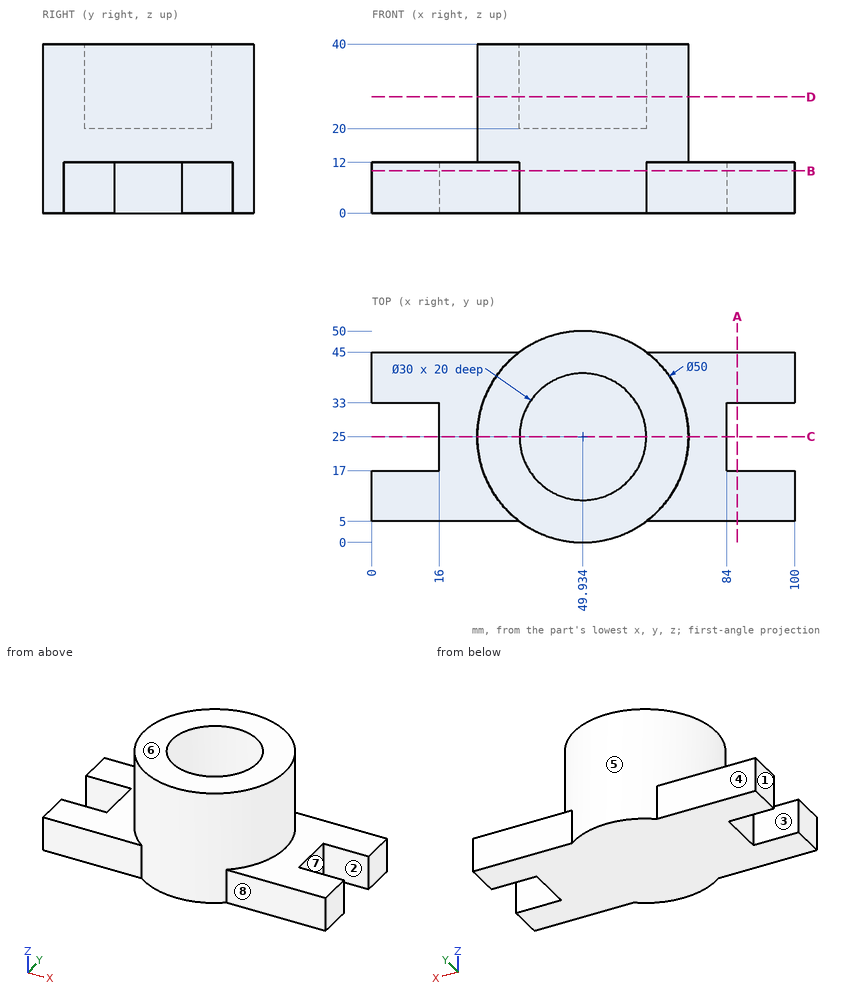
Check sheet for the drawn part. Datum: minimum x, y, z corner. Units: mm. A direction names the side the tool comes from. Coordinates: 2 decimals unless noted, no trailing zeros. Loops run counter-clockwise (first coordinate to the right, second up) from the corner with the lowest first, then second, coordinate; pieces in that order, holes last. Notation, with made-up numbers: (-33, 19) -> (15, 19) arc R16 ccw to (15, 44) -> close; hole circle Ø4 at (13.5, 10). An arc over 180 degrees is marked (long way). Answer as a JSON object with one key per item and string values. Group by question number.
Item 1: Scan lines: probe 1 along Y at (x, z) = (85.5, 9.5); probe 2 along X at (y, z) = (17.5, 8.5); probe 3 along Z at (x, y) = (23, 5.5). Record each from-to range of solid material in increasing order.
Item 2: Sectioned sample at A-A on x = 86.5. Record the boundary of the cut face in (y, z).
Item 3: Tool access check on the marked faces 1, 2, 3, 4 and 5. Record the directions out of +Z, -Z, +X, -X, +Y, -Y that give a thin tool (end or side, any length) a straight path to the whole face; none if there is none.
Item 4: Sectioned sample at D-D on z = 27.5. Record the boundary of the cut face in (x, y).
Item 5: Depth check by flat-ended pin: pin 1 (9.5 mm diameter, centred on x = 91.5, z = 8.5, fed in from +Y); pin 2 (24 mm diameter, centred on x = 49.93, y = 25, fed in from +Z); pin 3 (9.5 mm diameter, centred on x = 85, z = 5.5, fed in from -Y). Enter the tip coordinate at first touch or a pass-through.
Item 6: Mould release check, pull along Y, two halves, no side actions. Record for the marked faces 6, 7 and 8: +Y half, -Y half, draft (parallel to the pull), parting line (faces both ways), or undercut.
Item 7: Sectioned sample at B-B on z = 10. Record the boundary of the cut face in (x, y), plus the area to 3 significant figures.
Item 8: Sectioned sample at C-C on y = 25. Record the boundary of the cut face in (x, z), plus the area to 3 significant figures.
Evaluation:
{
 "1": {"probe 1": "y = 5 to 17, 33 to 45", "probe 2": "x = 16 to 84", "probe 3": "z = 0 to 12"},
 "2": {"outline": "(5, 0) -> (17, 0) -> (17, 12) -> (5, 12) -> close; (33, 0) -> (45, 0) -> (45, 12) -> (33, 12) -> close"},
 "3": {"face 1": "+Z, -Z, -X, +Y, -Y", "face 2": "+Z, -Z, +X", "face 3": "+Z, -Z, -X", "face 4": "+Z, -Z, -X, +Y", "face 5": "+Z"},
 "4": {"outline": "circle Ø50 at (49.93, 25); hole circle Ø30 at (49.93, 25)"},
 "5": {"pin 1": "stops at y = 45", "pin 2": "stops at z = 20", "pin 3": "stops at y = 5"},
 "6": {"face 6": "draft", "face 7": "undercut", "face 8": "-Y half"},
 "7": {"outline": "(0, 5) -> (34.93, 5) arc R25 ccw to (64.93, 5) -> (100, 5) -> (100, 17) -> (84, 17) -> (84, 33) -> (100, 33) -> (100, 45) -> (64.93, 45) arc R25 ccw to (34.93, 45) -> (0, 45) -> (0, 33) -> (16, 33) -> (16, 17) -> (0, 17) -> close", "area": "3,690 mm²"},
 "8": {"outline": "(16, 0) -> (84, 0) -> (84, 12) -> (74.93, 12) -> (74.93, 40) -> (64.93, 40) -> (64.93, 20) -> (34.93, 20) -> (34.93, 40) -> (24.93, 40) -> (24.93, 12) -> (16, 12) -> close", "area": "1,620 mm²"}
}
